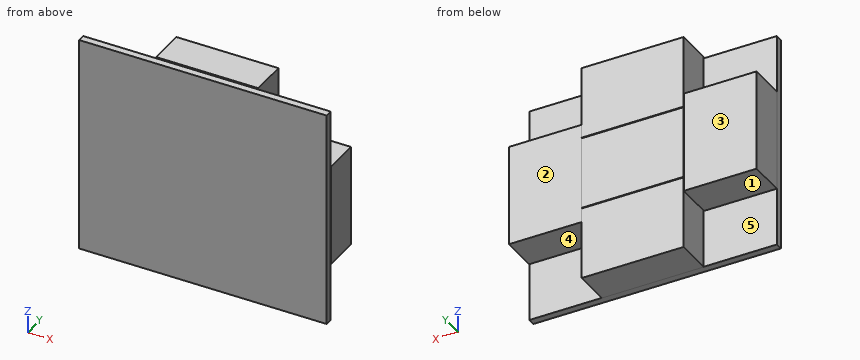
```python
from build123d import *

# Parameters (mm, degrees)
SKETCH1_W           = 170
SKETCH1_H           = 150
BOSS_EXTRUDE1_DEPTH = 5
SKETCH4_W           = 65
SKETCH4_H           = 45
BOSS_EXTRUDE2_DEPTH = 0.5
SKETCH5_W           = 70
SKETCH5_H           = 50.044144688
BOSS_EXTRUDE3_DEPTH = 25
LPATTERN3_COUNT     = 2
LPATTERN3_PITCH     = 50.5
LPATTERN3_COL_COUNT = 2
LPATTERN3_COL_PITCH = 50.5
SKETCH6_W           = 45
SKETCH6_H           = 65
BOSS_EXTRUDE4_DEPTH = 0.2
SKETCH7_W           = 50
SKETCH7_H           = 70
BOSS_EXTRUDE5_DEPTH = 25
LPATTERN4_COUNT     = 2
LPATTERN4_PITCH     = 120


with BuildPart() as part:
    # Sketch1 → Boss-Extrude1 (new body)
    with BuildSketch(Plane(origin=(0, 0, 0), x_dir=(1, 0, 0), z_dir=(0, 1, 0))):
        Rectangle(SKETCH1_W, SKETCH1_H)
    extrude(amount=BOSS_EXTRUDE1_DEPTH)

    # Sketch4 → Boss-Extrude2 (add)
    with BuildSketch(Plane(origin=(0, 5, 0), x_dir=(1, 0, 0), z_dir=(0, 1, 0))):
        Rectangle(SKETCH4_W, SKETCH4_H)
    boss_extrude2 = extrude(amount=BOSS_EXTRUDE2_DEPTH)

    # Sketch5 → Boss-Extrude3 (add)
    with BuildSketch(Plane(origin=(0, 5.5, 0), x_dir=(1, 0, 0), z_dir=(0, 1, 0))):
        Rectangle(SKETCH5_W, SKETCH5_H)
    boss_extrude3 = extrude(amount=BOSS_EXTRUDE3_DEPTH)

    # LPattern3: Boss-Extrude2, Boss-Extrude3 ×2
    with Locations(*[(0, 0, i * LPATTERN3_PITCH) for i in range(1, LPATTERN3_COUNT)]):
        add(boss_extrude2)
        add(boss_extrude3)

    # LPattern3 col: Boss-Extrude2, Boss-Extrude3 ×2
    with Locations(*[(0, 0, -i * LPATTERN3_COL_PITCH) for i in range(1, LPATTERN3_COL_COUNT)]):
        add(boss_extrude2)
        add(boss_extrude3)

    # Sketch6 → Boss-Extrude4 (add)
    with BuildSketch(Plane(origin=(0, 5, 0), x_dir=(1, 0, 0), z_dir=(0, 1, 0))):
        with Locations((60, 0)):
            Rectangle(SKETCH6_W, SKETCH6_H)
    boss_extrude4 = extrude(amount=BOSS_EXTRUDE4_DEPTH)

    # Sketch7 → Boss-Extrude5 (add)
    with BuildSketch(Plane(origin=(0, 5.2, 0), x_dir=(1, 0, 0), z_dir=(0, 1, 0))):
        with Locations((60, 0)):
            Rectangle(SKETCH7_W, SKETCH7_H)
    boss_extrude5 = extrude(amount=BOSS_EXTRUDE5_DEPTH)

    # LPattern4: Boss-Extrude4, Boss-Extrude5 ×2
    with Locations(*[(-i * LPATTERN4_PITCH, 0, 0) for i in range(1, LPATTERN4_COUNT)]):
        add(boss_extrude4)
        add(boss_extrude5)


solid = part.part
```
For this review, take the finished solid that the model builds, in its own axes (mm). Face numbers are marked on the shaded views. A direction names the side the tool comes from. Round coordinates to 2 decimals unless told otherwise and drop trailing zeros. Write each loop counter-clockwise with the first axis right and the second up, starting at its lowest first coordinate (ties: lowest second). Pieces come first, ordered by that corner, then holes. Notation, with made-up numbers: (72, -18.75) -> (110, -18.75) arc R33 ccw to (110, 19.25) -> close; hole circle Ø8 at (55, -12). An arc over 180 degrees is marked (long way). One line per question, with ' | ' between items. Start each with the question number.
1) Machinability: for the marked faces 1, 2, 3, 4 and 5, which of the approach directions +Z, -Z, +X, -X, +Y, -Y give a long, thin tool a straight path to every point of the face, cutting with its end or side? Answer none if there is none.
2) Add section B-B (y = 12.5). Write out the cut boundary in (x, z), and give its area (3 significant figures).
3) Add section A-A (x = -62). Write out the cut boundary in (y, z), and give its area (3 significant figures).
4) Wall thickness on line 1 along Z through (x, y) = (12.5, 8); line 2 along Y through (x, z) = (-50, 21.5); line 3 along Z through (x, y) = (68, 17): over which ranges is each line inside the solid? List them lowest first.
5) Add section C-C (z = 60). Write out the cut boundary in (x, y).
6) For pin 1 Ø12.5 at (x, y) = (54.5, 16.5) entering from +Z; pin 2 Ø4 at (x, y) = (54.5, 12) entering from -Z; pin 3 Ø1 at (x, z) = (57, 34.5) entering from +Y, all flat-tipped, find the tip position at first contact; note any pin that passes through.
Reported:
1) face 1: -Z, -X, +Y | face 2: +Z, -Z, +X, +Y | face 3: +Z, -Z, -X, +Y | face 4: -Z, +X, +Y | face 5: none
2) outline: (-85, -35) -> (-35, -35) -> (-35, -75.52) -> (35, -75.52) -> (35, -35) -> (85, -35) -> (85, 35) -> (35, 35) -> (35, 75.52) -> (-35, 75.52) -> (-35, 35) -> (-85, 35) -> close; hole (-35, -25.48) -> (35, -25.48) -> (35, -25.02) -> (-35, -25.02) -> close; hole (-35, 25.02) -> (35, 25.02) -> (35, 25.48) -> (-35, 25.48) -> close | area: 17,500 mm²
3) outline: (0, -75) -> (5, -75) -> (5, -32.5) -> (5.2, -32.5) -> (5.2, -35) -> (30.2, -35) -> (30.2, 35) -> (5.2, 35) -> (5.2, 32.5) -> (5, 32.5) -> (5, 75) -> (0, 75) -> close | area: 2,510 mm²
4) line 1: z = -75.52 to -25.48, -25.02 to 25.02, 25.48 to 75.52 | line 2: y = 0 to 30.2 | line 3: z = -35 to 35
5) outline: (-85, 0) -> (85, 0) -> (85, 5) -> (32.5, 5) -> (32.5, 5.5) -> (35, 5.5) -> (35, 30.5) -> (-35, 30.5) -> (-35, 5.5) -> (-32.5, 5.5) -> (-32.5, 5) -> (-85, 5) -> close
6) pin 1: stops at z = 35 | pin 2: stops at z = -35 | pin 3: stops at y = 30.2
